Could you check a few things on this model? Use its own coordinates, in mm. Face numbers are marked on the shaded views. A direction names the side the tool comes from. Coordinates: 2 decimals unless noted, no trailing zeros. Loops run counter-clockwise (first coordinate to the right, second up) from the corner with the lowest first, then second, coordinate; pieces in that order, holes last. Notation, with made-up numbers: M -5.75,43 L 33.25,43 A21 ccw 33.25,58 Z; hole C 79.5,-37 d11. An arc over 180 degrees is marked long. Write each question's results on one line, items separated by ' | '.
```python
from build123d import *

# Parameters (mm, degrees)
ESQUISSE2_R             = 1.5
ENL_V_MAT_EXTRU_1_DEPTH = 7.5
ESQUISSE3_R             = 19.4
ENL_V_MAT_EXTRU_2_DEPTH = 14.5


with BuildPart() as part:
    # Esquisse1 → Révolution1 (revolve)
    with BuildSketch(Plane.XY, mode=Mode.PRIVATE) as r_volution1_sk:
        Polygon((0, 20.9), (14.32, 20.9), (19.32, 10), (19.32, 2), (24.12, 2), (24.12, 0), (0, 0), align=None)
    revolve(r_volution1_sk.sketch.rotate(Axis((0, 0, 0), (1, 0, 0)), 90), axis=Axis((0, 0, 0), (1, 0, 0)))

    # Esquisse2 → Enlèv. mat.-Extru.1 (cut)
    with BuildSketch(Plane(origin=(19.32, 0, 0), x_dir=(0, 0, -1), z_dir=(1, 0, 0))):
        with Locations(Location((0, -5.66, 0), (0, 0, 180))):
            Circle(ESQUISSE2_R)
        with Locations((-5.66, 0)):
            Circle(ESQUISSE2_R)
        with Locations(Location((0, 5.66, 0), (0, 0, 180))):
            Circle(ESQUISSE2_R)
        with Locations((5.66, 0)):
            Circle(ESQUISSE2_R)
    extrude(amount=-ENL_V_MAT_EXTRU_1_DEPTH, mode=Mode.SUBTRACT)

    # Esquisse3 → Enlèv. mat.-Extru.2 (cut)
    with BuildSketch(Plane.ZY):
        Circle(ESQUISSE3_R)
    extrude(amount=-ENL_V_MAT_EXTRU_2_DEPTH, mode=Mode.SUBTRACT)


solid = part.part
```
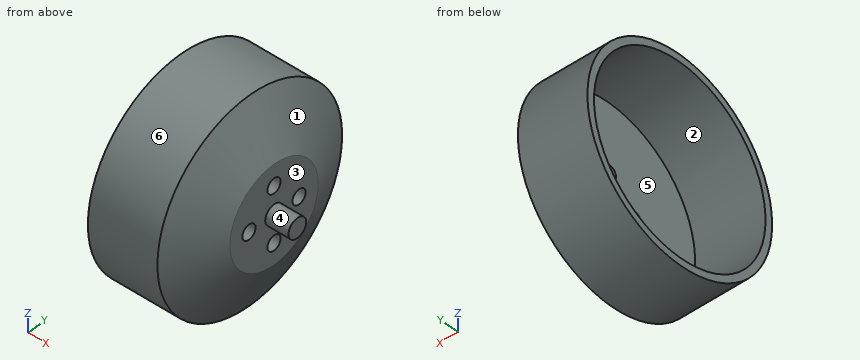
(1) If we mould it in two halves opening along Z, with no side actions, what happens to the marked faces 1, 2 and 3? For each: released by +Z, released by -Z, zero draft, split by the parting line, or undercut.
Reported:
face 1: split by the parting line | face 2: undercut | face 3: zero draft
(2) Will these pins go through, and if not, where does the flat tip stop? P1, Ø1.5, axis at y = 15.5, z = 0.5, coming from the +X side; P2, Ø8, axis at x = 9, y = -7.5, coming from the +Z side; P3, Ø2, axis at x = 15.5, z = 7, coming from the +Y side.
Reported:
P1: stops at x = 17.14 | P2: stops at z = 20.6 | P3: stops at y = 19.3
(3) Please list where these lines run through material, in increasing order: probe 1 along Y at (x, z) = (18.35, 0); probe 2 along Y at (x, z) = (17.9, 0); probe 3 along Z at (x, y) = (11.75, 5). Write a range as from..to.
Reported:
probe 1: y = -12.11..-7.16, -4.16..4.16, 7.16..12.11 | probe 2: y = -13.1..-7.16, -4.16..4.16, 7.16..13.1 | probe 3: z = -20.29..-18.74, 18.74..20.29
(4) Imagine slicing it at D-D, the plane x = 18.75. List the corners of the cut face in (y, z) for me.
Reported:
outline: C 0,0 d22.49; hole C -5.66,0 d3; hole C 0,-5.66 d3; hole C 0,5.66 d3; hole C 5.66,0 d3
(5) Which directions (+Z, -Z, +X, -X, +Y, -Y) give clear straight access to the entire face, cutting with the end or side of a thin tool? Please do the marked faces 4, 5 and 6.
Reported:
face 4: +X | face 5: -X | face 6: +X, -X
(6) Imagine slicing it at A-A, the plane y = 0. List the corners of the cut face in (x, z) for me.
Reported:
outline: M 0,-20.9 L 14.32,-20.9 L 19.32,-10 L 19.32,-7.16 L 14.5,-7.16 L 14.5,-19.4 L 0,-19.4 Z; M 0,19.4 L 14.5,19.4 L 14.5,7.16 L 19.32,7.16 L 19.32,10 L 14.32,20.9 L 0,20.9 Z; M 14.5,-4.16 L 19.32,-4.16 L 19.32,-2 L 24.12,-2 L 24.12,2 L 19.32,2 L 19.32,4.16 L 14.5,4.16 Z
(7) Imagine slicing it at C-C, the plane x = 16. List the corners of the cut face in (y, z) for me.
Reported:
outline: C 0,0 d34.48; hole C -5.66,0 d3; hole C 0,-5.66 d3; hole C 0,5.66 d3; hole C 5.66,0 d3
